Verification items for the finished model (mm, model axes). A direction names the side the tool comes from. Give positions to 0.01 mm unless a question says otherwise; leave off trailing zeros. Write each loop counter-clockwise with the first axis right and the second up, starting at its lowest first coordinate (ties: lowest second). Pieces come first, ordered by that corner, then holes. Notation, with made-up numbers: (-3.5, -20.5) -> (9.5, -20.5) arc R25 cw to (9.5, -6.5) -> close; hole circle Ø4 at (42, 52.5). An arc over 180 degrees is marked (long way). Use CSV: the item, a comma, the result in double quotes. Start each with the question number.
Autodesk Inventor part; units mm, degrees
ref_plane "YZ Plane" through (0, 0, 0) normal (1, 0, 0) x (0, 1, 0)
ref_plane "XZ Plane" through (0, 0, 0) normal (0, 1, 0) x (-1, 0, 0)
ref_plane "XY Plane" through (0, 0, 0) normal (0, 0, 1) x (1, 0, 0)
sketch "Sketch1" plane through (0, 0, 0) normal (0, 1, 0) x (-1, 0, 0)
  line L0 (0, 0) -> (-25.4, 0)
  line L1 (-25.4, 0) -> (-25.4, -25.4)
  line L2 (-25.4, -25.4) -> (0, -25.4)
  line L3 (0, -25.4) -> (0, 0)
  line L4 (0, 0) -> (-25.4, -25.4) construction
  line L5 (0, -25.4) -> (-25.4, 0) construction
  circle A0 centre (-12.7, -12.7) radius 3.175
  dimension "d0" = 25.4
  dimension "d1" = 25.4
  dimension "d3" = 6.35
extrude "Extrusion1" add sketch "Sketch1" along normal blind 25.4
sketch "Sketch2" plane through (0, 25.4, 0) normal (0, 1, 0) x (1, 0, 0)
  circle A0 centre (12.689, 12.689) radius 9.525
  point P0 (0, 0)
  dimension "d6" = 19.05
extrude "Extrusion2" cut sketch "Sketch2" against normal blind 3.175
sketch "Sketch3" plane through (0, 0, 0) normal (0, -1, 0) x (1, 0, 0)
  circle A0 centre (12.689, -12.689) radius 9.525
  circle A1 centre (12.689, -12.689) radius 9.525
  point P0 (0, 0)
  dimension "d9" = 19.05
extrude "Extrusion3" cut sketch "Sketch3" against normal blind 3.175
properties part number "MountingBracket_3"
(1) Section check C-C on x = 7.5. Record the cut outline in (y, z) (3 decimals).
(2) Section check B-B on y = 4.25. Record the cut outline in (x, z) (3 decimals).
(3) Go/stop test with flat-tipped pins: pin 1 (7.5 mm diameter, centred on x = 12.7, z = -12.7, fed in from +Y) (3 decimals); pin 2 (6 mm diameter, centred on x = 3.5, y = 20, fed in from +Z). Record where each tip stops, or that it passes through.
(4) Set-up check for faces 4 (the face through (5.13, 1.565, -18.485)), 5 (the face through (7, 25.4, -4)), 6 (the face through (10, 22.225, -15)): record each of +Z, -Z, +X, -X, +Y, -Y from which the full face is reachable in a straight line by a thin tool's end or side.
(5) Section check A-A on x = 12.7. Record the cut outline in (y, z) (3 decimals), then the cut area to 3 significant figures.
(6) Draft check along Z on faces 1 (the face through (0, 13, -13)), 2 (the face through (13, 13, -25.4)), 3 (the face through (5.67, 23.83, -19.13)). Enter one of: released by +Z, released by -Z, zero draft, split by the parting line, or undercut.
(7) Thickness scan on line 1 (X direction, y = 8, z = -12.5); line 2 (Z direction, x = 12.7, y = 11.75) (3 decimals); line 3 (Z direction, x = 13, y = 22.75). Record the ranges inside material, lowest first. Write a range as from..to.
(8) Section check D-D on z = -20.75. Record the cut outline in (x, y) (3 decimals).
Data:
1,outline,"(0, -25.4) -> (25.4, -25.4) -> (25.4, -20.676) -> (22.225, -20.676) -> (22.225, -4.702) -> (25.4, -4.702) -> (25.4, 0) -> (0, 0) -> (0, -4.702) -> (3.175, -4.702) -> (3.175, -20.676) -> (0, -20.676) -> close"
2,outline,"(0, -25.4) -> (25.4, -25.4) -> (25.4, 0) -> (0, 0) -> close; hole circle Ø6.35 at (12.7, -12.7)"
3,pin 1,"stops at y = 22.225"
3,pin 2,"stops at z = 0"
4,face 4,"-Y"
4,face 5,"+Z, -Z, +X, -X, +Y"
4,face 6,"+Y"
5,outline,"(0, -25.4) -> (25.4, -25.4) -> (25.4, -22.214) -> (22.225, -22.214) -> (22.225, -15.875) -> (3.175, -15.875) -> (3.175, -22.214) -> (0, -22.214) -> close; (0, -3.164) -> (3.175, -3.164) -> (3.175, -9.525) -> (22.225, -9.525) -> (22.225, -3.164) -> (25.4, -3.164) -> (25.4, 0) -> (0, 0) -> close"
5,area,"403 mm2"
6,face 1,"zero draft"
6,face 2,"released by -Z"
6,face 3,"undercut"
7,line 1,"x = 0..9.53, 15.87..25.4"
7,line 2,"z = -25.4..-15.875, -9.525..0"
7,line 3,"z = -25.4..-22.21, -3.17..0"
8,outline,"(0, 0) -> (7.615, 0) -> (7.615, 3.175) -> (17.763, 3.175) -> (17.763, 0) -> (25.4, 0) -> (25.4, 25.4) -> (17.763, 25.4) -> (17.763, 22.225) -> (7.615, 22.225) -> (7.615, 25.4) -> (0, 25.4) -> close"
